```python
from build123d import *

# Parameters (mm, degrees)
SALIENTE_EXTRUIR2_DEPTH = 200
CORTAR_EXTRUIR1_START   = -22
CROQUIS2_R              = 6.238263744
CROQUIS2_R_2            = 6.628155228
CORTAR_EXTRUIR1_DEPTH   = 22
CHAFL_N1_SIZE           = 2
CHAFL_N2_SIZE           = 5


with BuildPart() as part:
    # Croquis1 → Saliente-Extruir2 (new body)
    with BuildSketch(Plane(origin=(0, 0, 0), x_dir=(1, 0, 0), z_dir=(0, 1, 0))):
        with BuildLine():
            Line((-110, 90), (110, 90))
            ThreePointArc((110, 90), (117.071067812, 87.071067812), (120, 80))
            Line((120, 80), (120, -80))
            ThreePointArc((120, -80), (117.071067812, -87.071067812), (110, -90))
            Line((110, -90), (-110, -90))
            ThreePointArc((-110, -90), (-117.071067812, -87.071067812), (-120, -80))
            Line((-120, -80), (-120, 80))
            ThreePointArc((-120, 80), (-117.071067812, 87.071067812), (-110, 90))
        make_face()
    extrude(amount=SALIENTE_EXTRUIR2_DEPTH)

    # Croquis2 → Cortar-Extruir1 (cut)
    # profile 1 of 2: a face of its own
    with BuildSketch(Plane(origin=(0, 200, 0), x_dir=(1, 0, 0), z_dir=(0, 1, 0)).offset(CORTAR_EXTRUIR1_START)):
        with BuildLine():
            Line((-120, 80), (-120, 41.298746549))
            Line((-120, 41.298746549), (120, 41.298746549))
            Line((120, 41.298746549), (120, 80))
            ThreePointArc((120, 80), (117.071067812, 87.071067812), (110, 90))
            Line((110, 90), (-110, 90))
            ThreePointArc((-110, 90), (-117.071067812, 87.071067812), (-120, 80))
        make_face()
    # profile 2 of 2: a face of its own
    with BuildSketch(Plane(origin=(0, 200, 0), x_dir=(1, 0, 0), z_dir=(0, 1, 0)).offset(CORTAR_EXTRUIR1_START)):
        with BuildLine():
            Line((-37.579902073, -26.031911332), (-120, -26.031911332))
            Line((-120, -26.031911332), (-120, -80))
            ThreePointArc((-120, -80), (-117.071067812, -87.071067812), (-110, -90))
            Line((-110, -90), (110, -90))
            ThreePointArc((110, -90), (117.071067812, -87.071067812), (120, -80))
            Line((120, -80), (120, -26.031911332))
            Line((120, -26.031911332), (52.063822663, -26.031911332))
            Line((52.063822663, -26.031911332), (52.063822663, -80))
            Line((52.063822663, -80), (-37.579902073, -80))
            Line((-37.579902073, -80), (-37.579902073, -26.031911332))
        make_face()
        with Locations(Location((-81.424491258, -57.813449816, 0), (0, 0, 270))):
            Circle(CROQUIS2_R, mode=Mode.SUBTRACT)
        with Locations(Location((88.958087252, -57.813449816, 0), (0, 0, 270))):
            Circle(CROQUIS2_R_2, mode=Mode.SUBTRACT)
    extrude(amount=CORTAR_EXTRUIR1_DEPTH, mode=Mode.SUBTRACT)

    # Chaflán1
    chafl_n1_edges = [part.edges().sort_by_distance(p)[0] for p in [
        (-81.424491258, 200, 51.575186072),
        (88.958087252, 200, 51.185294588),
    ]]
    chamfer(chafl_n1_edges, length=CHAFL_N1_SIZE)

    # Chaflán2
    chafl_n2_edges = [part.edges().sort_by_distance(p)[0] for p in [
        (-120, 200, -7.633417609),
        (0, 200, -41.298746549),
        (120, 200, -7.633417609),
        (52.063822663, 200, 53.015955666),
        (-37.579902073, 200, 53.015955666),
        (7.241960295, 200, 80),
        (-78.789951036, 200, 26.031911332),
        (86.031911332, 200, 26.031911332),
    ]]
    chamfer(chafl_n2_edges, length=CHAFL_N2_SIZE)


solid = part.part
```
Read the model definition and answer for the solid it produces. Units are mm, in the model's axes. A direction names the side the tool comes from. Give positions to 0.01 mm unless a question says otherwise; leave off trailing zeros. Loops run counter-clockwise (first coordinate to the right, second up) from the corner with the lowest first, then second, coordinate; pieces in that order, holes last.
Item 1: The part is cut by section B-B (z = 36). Write down the section's boundary in (x, y).
Item 2: The part is cut by section A-A (x = 12). Write down the section's boundary in (y, z), and give its area (3 significant figures).
Item 3: Each of these flat-tipped pins is pushed along its axis until it touches: pin 1 Ø1.5 at (x, z) = (57, 39.5) entering from +Y; pin 2 Ø8.5 at (y, z) = (183.5, 49.5) entering from -X; pin 3 Ø5 at (x, y) = (78.5, 185.5) entering from +Z. Where does it stop, or does it pass through?
Item 4: Find the intervals of material crossed by line 1 along Y through (x, z) = (-90.5, -66); line 2 along Z through (x, y) = (-35, 185); line 3 along X through (y, z) = (123, -81), in increasing order.
Item 5: For faces 4 (the flat face through (-78, 186, 26.032)), 5 (the cylindrical face through (-117.15, 87.75, -86.99)), 6 (the flat face through (8, 186, 80)), 7 (the cylindrical face through (116.99, 87.75, -87.15)), 8 (the flat face through (-37.58, 186, 53)), determine the directions among +Z, -Z, +X, -X, +Y, -Y from which every point of the face is accessible in a straight line to the end or side of a thin tool.
Item 6: The mould has two halves that part along Z. Classify faces 1 (the cylindrical face through (95.53, 187.86, 56.95)), 2 (the flat face through (-81, 200, 58)), 3 (the flat face through (-2, 186, -41.299)): released by +Z, released by -Z, zero draft, split by the parting line, or undercut.
Taken from the geometry:
1. outline: (-120, 0) - (120, 0) - (120, 178) - (52.06, 178) - (52.06, 195) - (47.06, 200) - (-32.58, 200) - (-37.58, 195) - (-37.58, 178) - (-120, 178) - close
2. outline: (0, -90) - (178, -90) - (178, -41.3) - (195, -41.3) - (200, -36.3) - (200, 75) - (195, 80) - (178, 80) - (178, 90) - (0, 90) - close
2. area: 34,700 mm2
3. pin 1: stops at y = 178
3. pin 2: stops at x = -86.16
3. pin 3: stops at z = 26.03
4. line 1: y = 0 to 178
4. line 2: z = -41.3 to 80
4. line 3: x = -119.95 to 119.95
5. face 4: -X, +Y
5. face 5: -Z, -X, +Y, -Y
5. face 6: +Z, +X, -X, +Y
5. face 7: -Z, +X, +Y, -Y
5. face 8: +Z, +Y
6. face 1: undercut
6. face 2: zero draft
6. face 3: released by -Z
